Can you work these out from the model? Positions are in its coordinate system, mm. Face numbers are marked on the shaded views. A direction names the side the tool comes from. Give positions to 0.01 mm unless a question says otherwise; leave off trailing zeros. Loops run counter-clockwise (first coordinate to the right, second up) from the corner with the lowest first, then second, coordinate; pieces in that order, holes last. Notation, with made-up numbers: M -14,-31.75 L 7,-31.75 A15 ccw 7,-27.75 Z; hole C 71,64 d10. An arc over 180 degrees is marked long. Put each result on its own line as item: value. Start each with the question number.
1) Imagine slicing it at D-D (z = 18). Write out the boundary of the cut face in (x, y), then the cut area to 3 significant figures.
2) If we mould it in two halves opening along Z, with no side actions, what happens to the marked faces 3, 4 and 5? For each: +Z half, -Z half, draft (parallel to the pull), parting line (faces both ways), or undercut.
3) For the marked faces 1 and 2, which set-ups out of +Z, -Z, +X, -X, +Y, -Y let a thin tool reach every point of the face, with its end or its side?
4) Please list where these lines run through material, in increasing order: line 1 along X through (y, z) = (13.5, 23.8); line 2 along Y through (x, z) = (46.55, 10); line 3 along Z through (x, y) = (-59, 19). Write a range as from..to.
5) For P1, Ø5, axis at y = 25.5, z = 10.5, coming from the +X side; P2, Ø3, axis at y = -9, z = 19.5, coming from the +X side; P3, Ø8, axis at x = -7, y = 33, coming from the +Z side; P4, Ø12, axis at y = 2.5, z = 25, coming from the -X side, each with a flat end and sliding along its axis, tell me the tip position at first contact or that it passes through.
6) Imagine slicing it at B-B (y = 22). Write out the boundary of the cut face in (x, z).
7) Imagine slicing it at C-C (z = 29.5). Write out the boundary of the cut face in (x, y).
8) Imagine slicing it at A-A (x = 81). Write out the boundary of the cut face in (y, z).
from build123d import *

# Parameters (mm, degrees)
EXTRUDE_1_DEPTH      = 5
SKETCH_2_W           = 5
SKETCH_2_H           = 25
EXTRUDE_2_DEPTH      = 10
SKETCH_3_R           = 1.5
CUT_EXTRUDE_1_DEPTH  = 120
FILLET_1_R           = 4
SKETCH_4_W           = 5
SKETCH_4_H           = 16
EXTRUDE_3_DEPTH      = 15
FILLET_3_R           = 7.5
EXTRUDE_4_DEPTH      = 10
EXTRUDE_4_DEPTH_BACK = 60
SKETCH_5_R           = 12.5
FILLET_4_R           = 12.5
SKETCH_6_R           = 1
EXTRUDE_5_DEPTH      = 10
SKETCH_7_R           = 1.6
CUT_EXTRUDE_2_DEPTH  = 40
CUT_EXTRUDE_START    = -40
SKETCH_8_R           = 1.6
CUT_EXTRUDE_3_DEPTH  = 40


with BuildPart() as part:
    # 草图1 → 凸台-拉伸1 (new body)
    with BuildSketch(Plane.XY):
        Polygon((-45.482044199, 8.198895028), (49.017955801, 8.198895028), (49.017955801, 18.198895028), (54.017955801, 18.198895028), (54.017955801, 8.198895028), (101.767955801, 8.198895028), (101.767955801, 33.198895028), (-98.232044199, 33.198895028), (-98.232044199, 8.198895028), (-50.482044199, 8.198895028), (-50.482044199, 18.198895028), (-45.482044199, 18.198895028), align=None)
    extrude(amount=EXTRUDE_1_DEPTH)

    # 草图2 → 凸台-拉伸2 (add)
    with BuildSketch(Plane.XY.offset(5)):
        with Locations((-42.982044199, 20.698895028)):
            Rectangle(SKETCH_2_W, SKETCH_2_H)
        with Locations((46.517955801, 20.698895028)):
            Rectangle(SKETCH_2_W, SKETCH_2_H)
    extrude(amount=EXTRUDE_2_DEPTH)

    # 草图3 → 切除-拉伸1 (cut)
    with BuildSketch(Plane(origin=(49.017955801, 0, 0), x_dir=(0, 0, -1), z_dir=(1, 0, 0))):
        with Locations((-10, 15.198895028)):
            Circle(SKETCH_3_R)
    extrude(amount=-CUT_EXTRUDE_1_DEPTH, mode=Mode.SUBTRACT)

    # 圆角1
    fillet_1_edges = [part.edges().sort_by_distance(p)[0] for p in [
        (-42.982044199, 8.198895028, 15),
        (-42.982044199, 33.198895028, 15),
        (46.517955801, 33.198895028, 15),
        (46.517955801, 8.198895028, 15),
    ]]
    fillet(fillet_1_edges, radius=FILLET_1_R)

    # 草图4 → 凸台-拉伸3 (add)
    with BuildSketch(Plane(origin=(0, 0, 0), x_dir=(-1, 0, 0), z_dir=(0, 0, -1))):
        with Locations((-104.267955801, 16.198895028)):
            Rectangle(SKETCH_4_W, SKETCH_4_H)
        with Locations((100.732044199, 16.198895028)):
            Rectangle(SKETCH_4_W, SKETCH_4_H)
    extrude(amount=-EXTRUDE_3_DEPTH)

    # 圆角3
    fillet_3_edges = [part.edges().sort_by_distance(p)[0] for p in [
        (-98.232044199, 16.198895028, 5),
        (-103.232044199, 16.198895028, 0),
        (101.767955801, 16.198895028, 5),
        (106.767955801, 16.198895028, 0),
    ]]
    fillet(fillet_3_edges, radius=FILLET_3_R)

    # 草图5 → 凸台-拉伸4 (add, two sides: drawn at the far end of the back side and taken through both)
    with BuildSketch(Plane(origin=(0, 33.198895028, 0), x_dir=(1, 0, 0), z_dir=(0, 1, 0)).offset(-EXTRUDE_4_DEPTH_BACK)):
        with Locations(Location((-109.232044199, -22, 0), (0, 0, 270))):
            Circle(SKETCH_5_R)
        with Locations(Location((112.767955801, -22, 0), (0, 0, 270))):
            Circle(SKETCH_5_R)
    extrude(amount=EXTRUDE_4_DEPTH + EXTRUDE_4_DEPTH_BACK)

    # 圆角4
    fillet_4_edges = [part.edges().sort_by_distance(p)[0] for p in [
        (-109.232044199, -26.801104972, 9.5),
        (112.767955801, -26.801104972, 9.5),
    ]]
    fillet(fillet_4_edges, radius=FILLET_4_R)

    # 草图6 → 凸台-拉伸5 (add)
    # profile 1 of 2: a face of its own
    with BuildSketch(Plane.XZ.offset(-8.198895028)):
        with BuildLine():
            ThreePointArc((89.017955801, 23.25), (97.267955801, 15), (89.017955801, 6.75))
            Line((89.017955801, 6.75), (83.802055385, 6.75))
            Line((83.802055385, 6.75), (83.802055385, 5))
            Line((83.802055385, 5), (104.017955801, 5))
            Line((104.017955801, 5), (104.017955801, 25))
            Line((104.017955801, 25), (54.017955801, 25))
            Line((54.017955801, 25), (54.017955801, 5))
            Line((54.017955801, 5), (70.296008778, 5))
            Line((70.296008778, 5), (70.296008778, 6.75))
            Line((70.296008778, 6.75), (64.017955801, 6.75))
            ThreePointArc((64.017955801, 6.75), (55.767955801, 15), (64.017955801, 23.25))
            Line((64.017955801, 23.25), (89.017955801, 23.25))
        make_face()
        with Locations(Location((55.217955801, 6.2, 0), (0, 0, 270))):
            Circle(SKETCH_6_R, mode=Mode.SUBTRACT)
        with Locations((96.217955801, 6.2)):
            Circle(SKETCH_6_R, mode=Mode.SUBTRACT)
        with Locations(Location((55.217955801, 23.8, 0), (0, 0, 270))):
            Circle(SKETCH_6_R, mode=Mode.SUBTRACT)
        with Locations(Location((96.217955801, 23.8, 0), (0, 0, 270))):
            Circle(SKETCH_6_R, mode=Mode.SUBTRACT)
    # profile 2 of 2: a face of its own
    with BuildSketch(Plane.XZ.offset(-8.198895028)):
        with BuildLine():
            Line((-66.760097176, 6.75), (-66.760097176, 5))
            Line((-66.760097176, 5), (-50.482044199, 5))
            Line((-50.482044199, 5), (-50.482044199, 25))
            Line((-50.482044199, 25), (-100.482044199, 25))
            Line((-100.482044199, 25), (-100.482044199, 5))
            Line((-100.482044199, 5), (-80.266143783, 5))
            Line((-80.266143783, 5), (-80.266143783, 6.75))
            Line((-80.266143783, 6.75), (-85.482044199, 6.75))
            ThreePointArc((-85.482044199, 6.75), (-93.732044199, 15), (-85.482044199, 23.25))
            Line((-85.482044199, 23.25), (-60.482044199, 23.25))
            ThreePointArc((-60.482044199, 23.25), (-52.232044199, 15), (-60.482044199, 6.75))
            Line((-60.482044199, 6.75), (-66.760097176, 6.75))
        make_face()
        with Locations((-92.682044199, 6.2)):
            Circle(SKETCH_6_R, mode=Mode.SUBTRACT)
        with Locations(Location((-51.682044199, 6.2, 0), (0, 0, 270))):
            Circle(SKETCH_6_R, mode=Mode.SUBTRACT)
        with Locations(Location((-92.682044199, 23.8, 0), (0, 0, 270))):
            Circle(SKETCH_6_R, mode=Mode.SUBTRACT)
        with Locations(Location((-51.682044199, 23.8, 0), (0, 0, 270))):
            Circle(SKETCH_6_R, mode=Mode.SUBTRACT)
    extrude(amount=-EXTRUDE_5_DEPTH)

    # 草图7 → 切除-拉伸2 (cut)
    with BuildSketch(Plane(origin=(-40.482044199, 0, 0), x_dir=(0, 0, -1), z_dir=(1, 0, 0))):
        with Locations((-10, 15.198895028)):
            Circle(SKETCH_7_R)
    extrude(amount=-CUT_EXTRUDE_2_DEPTH, mode=Mode.SUBTRACT)

    # 草图8 → 切除-拉伸3 (cut)
    with BuildSketch(Plane.ZY.offset(-44.017955801).offset(CUT_EXTRUDE_START)):
        with Locations(Location((10, 15.198895028, 0), (0, 0, 180))):
            Circle(SKETCH_8_R)
    extrude(amount=CUT_EXTRUDE_3_DEPTH, mode=Mode.SUBTRACT)


solid = part.part
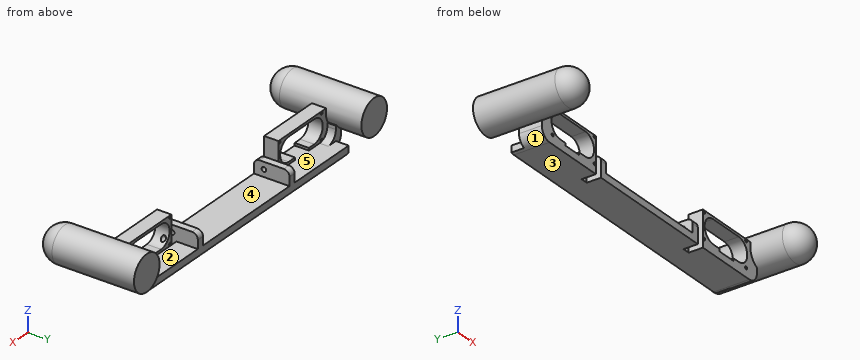
Recorded:
1. outline: M -121.07,-14.3 A11.84 ccw -97.39,-14.3 L -97.39,8.2 L -93.17,8.2 L -93.17,18.2 L -97.39,18.2 L -97.39,43.2 L -121.07,43.2 Z; M -52.8,8.2 L -50.48,8.2 L -50.48,18.2 L -52.8,18.2 Z; M 54.02,8.2 L 56.33,8.2 L 56.33,18.2 L 54.02,18.2 Z; M 96.7,8.2 L 100.93,8.2 L 100.93,-14.3 A11.84 ccw 124.61,-14.3 L 124.61,43.2 L 100.93,43.2 L 100.93,18.2 L 96.7,18.2 Z
1. area: 3,300 mm²
2. face 3: -Z half
2. face 4: +Z half
2. face 5: undercut
3. face 1: -Z, -X, +Y, -Y
3. face 2: +Y
4. line 1: -121.6..-93.68, -91.68..-52.68, -50.68..-50.48, 54.02..54.22, 56.22..95.22, 97.22..125.14
4. line 2: 8.2..13.6, 16.8..33.2
4. line 3: 0..5
5. P1: x = 121.44
5. P2: x = 125.23
5. P3: z = 5
5. P4: x = -121.73
6. outline: M -103.23,7.5 A7.5 ccw -95.73,0 L 99.27,0 A7.5 ccw 106.77,7.5 L 106.77,11.03 A12.5 ccw long 102.41,15 L 101.77,15 L 101.77,12.5 A7.5 cw 94.27,5 L 49.02,5 L 49.02,15 L 44.02,15 L 44.02,5 L -40.48,5 L -40.48,15 L -45.48,15 L -45.48,5 L -90.73,5 A7.5 cw -98.23,12.5 L -98.23,15 L -98.88,15 A12.5 ccw long -103.23,11.03 Z
7. outline: M -119.23,-14.3 A10 ccw -99.23,-14.3 L -99.23,43.2 L -119.23,43.2 Z; M 102.77,-14.3 A10 ccw 122.77,-14.3 L 122.77,43.2 L 102.77,43.2 Z
8. outline: M 8.2,0 L 33.2,0 L 33.2,5 L 8.2,5 Z; M 8.2,23.25 L 18.2,23.25 L 18.2,25 L 8.2,25 Z
